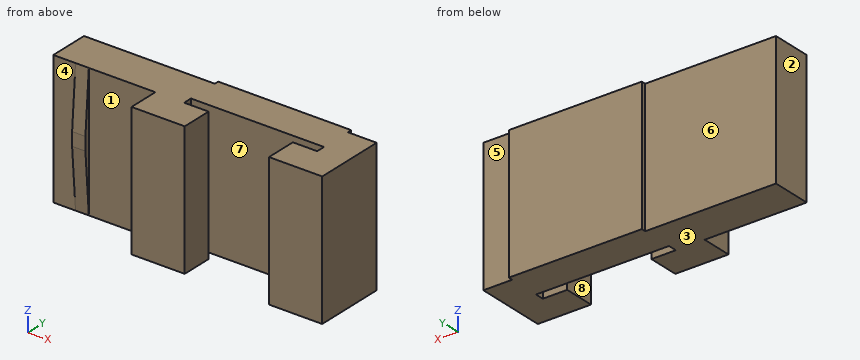
Autodesk Inventor part; units mm, degrees
ref_plane "YZ Plane" through (0, 0, 0) normal (1, 0, 0) x (0, 1, 0)
ref_plane "XZ Plane" through (0, 0, 0) normal (0, 1, 0) x (-1, 0, 0)
ref_plane "XY Plane" through (0, 0, 0) normal (0, 0, 1) x (1, 0, 0)
sketch "Skizze1" plane through (0, 0, 0) normal (0, 0, 1) x (1, 0, 0)
  line L0 (-41.25, -314) -> (-33.75, -314)
  line L1 (-41.25, -312) -> (-41.25, -314)
  line L2 (-11.25, -312) -> (-41.25, -312)
  line L3 (-18.75, -314) -> (-11.25, -314)
  line L4 (-11.25, -314) -> (-11.25, -312)
  line L5 (-18.75, -314) -> (-16.75, -314)
  line L6 (-16.75, -314) -> (-16.75, -321)
  line L7 (-16.75, -321) -> (-4.75, -321)
  line L8 (-4.75, -321) -> (-4.75, -305)
  line L9 (-4.75, -305) -> (-70.75, -305)
  line L10 (-70.75, -305) -> (-70.75, -314)
  line L11 (-47.75, -314) -> (-47.75, -321)
  line L12 (-47.75, -321) -> (-35.75, -321)
  line L13 (-35.75, -321) -> (-35.75, -314)
  line L14 (-35.75, -314) -> (-33.75, -314)
  line L15 (-70.75, -314) -> (-65.75, -314)
  line L16 (-65.75, -314) -> (-65.75, -315)
  line L17 (-65.75, -315) -> (-62.75, -315)
  line L18 (-62.75, -315) -> (-62.75, -314)
  line L19 (-62.75, -314) -> (-47.75, -314)
  line L20 (-26.25, -311) -> (-26.25, -312) construction
  point P0 (0, 0)
  point P1 (-64.25, -315)
  dimension "d0" = 2
  dimension "d1" = 7
  dimension "d2" = 12
  dimension "d3" = 16
  dimension "d4" = 12
  dimension "d5" = 2
  dimension "d6" = 3
  dimension "d7" = 38
  dimension "d8" = 5
  dimension "d9" = 1
extrude "Extrusion1" add sketch "Skizze1" along normal blind 30
chamfer "Fasen1" distance 1 distance2 13.5 1 edges at (-64.25, -315, 30) measured on face at (-38.9167, -307.3333, 30)
chamfer "Fasen2" distance 1 distance2 13.5 1 edges at (-64.25, -315, 0) measured on face at (-38.9167, -307.3333, 0)
sketch "Skizze2" plane through (-70.75, -305, 0) normal (0, 1, 0) x (1, 0, 0)
  line L0 (29.5, 0) -> (59.5, 0)
  line L1 (59.5, 0) -> (59.5, -30)
  line L2 (29.5, 0) -> (59.5, 0)
  line L3 (59.5, 0) -> (59.5, -30)
  line L4 (59.5, -30) -> (29.5, -30)
  line L5 (29.5, -30) -> (29.5, 0)
  point P0 (70.75, 0)
extrude "Extrusion2" add sketch "Skizze2" along normal blind 1
properties part number "KatzeFEM" material "Aluminium 6061, Katze"
Model file for the job. Use its own axes, mm. Face numbers are marked on the shaded views. A direction names the side the tool comes from. Give positions to 0.01 mm unless a question says otherwise; leave off trailing zeros. Loops run counter-clockwise (first coordinate to the right, second up) from the corner with the lowest first, then second, coordinate; pieces in that order, holes last. Notation, with made-up numbers: (-15.5, 72) - (40.5, 72) arc R30 ccw to (40.5, 107) - close; hole circle Ø7 at (-22.75, 8). An arc over 180 degrees is marked (long way). One line per item, written item: value. Start each with the question number.
1. Slice it at C-C (z = 15). List the corners of the cut face in (x, y).
2. Probe L1, parallel to X at y = -320, z = 5; L2, parallel to Y at x = -36, z = 21.5; L3, parallel to Y at x = -28, z = 3.5. List the from-to ranges inside material, lowest first. Write a range as from..to.
3. Slice it at B-B (x = -12.5). List the corners of the cut face in (y, z), plus the area to 3 significant figures.
4. Slice it at A-A (y = -316.75). List the corners of the cut face in (x, z), plus the area to 3 significant figures.
5. Which spindle directions (+Z, -Z, +X, -X, +Y, -Y) get a long thin tool onto all of the face, cutting with end or side? Do the marked faces 4, 5, 6, 7 and 8. Say none if no direction does.
6. Pull direction X, two halves, no side cores. Call the marked faces 1, 2 and 3: pulls with the +X half, pulls with the -X half, needs draft (parallel to the pull), parting line crosses it, or undercut.
7. Slice it at D-D (x = -21.5). List the corners of the cut face in (y, z), plus the area to 3 significant figures.
8. Pin check, flat tips, straight feed: pin 1 (1.5 mm diameter, centred on x = -69, z = 13.5, fed in from -Y); pin 2 (5 mm diameter, centred on x = -28, y = -315.5, fed in from -Z); pin 3 (5 mm diameter, centred on x = -7, z = 12.5, fed in from +Y); pin 4 (2 mm diameter, centred on y = -319, z = 22.5, fed in from -X). Stop position of each tip, or through.
Solution:
1. outline: (-70.75, -314) - (-65.75, -314) - (-65.75, -315) - (-62.75, -315) - (-62.75, -314) - (-47.75, -314) - (-47.75, -321) - (-35.75, -321) - (-35.75, -314) - (-41.25, -314) - (-41.25, -312) - (-11.25, -312) - (-11.25, -314) - (-16.75, -314) - (-16.75, -321) - (-4.75, -321) - (-4.75, -305) - (-11.25, -305) - (-11.25, -304) - (-41.25, -304) - (-41.25, -305) - (-70.75, -305) - close
2. L1: x = -47.75..-35.75, -16.75..-4.75
2. L2: y = -321..-314, -312..-304
2. L3: y = -312..-304
3. outline: (-321, 0) - (-314, 0) - (-314, 30) - (-321, 30) - close; (-312, 0) - (-304, 0) - (-304, 30) - (-312, 30) - close
3. area: 450 mm^2
4. outline: (-47.75, 0) - (-35.75, 0) - (-35.75, 30) - (-47.75, 30) - close; (-16.75, 0) - (-4.75, 0) - (-4.75, 30) - (-16.75, 30) - close
4. area: 720 mm^2
5. face 4: +Z, -Z, -X, -Y
5. face 5: +Z, -Z, +X, +Y
5. face 6: +Z, -Z, -X, +Y
5. face 7: +Z, -Z
5. face 8: +Z, -Z, -Y
6. face 1: undercut
6. face 2: pulls with the -X half
6. face 3: needs draft
7. outline: (-312, 0) - (-304, 0) - (-304, 30) - (-312, 30) - close
7. area: 240 mm^2
8. pin 1: stops at y = -314
8. pin 2: passes through
8. pin 3: stops at y = -305
8. pin 4: stops at x = -47.75
